Check sheet for the modelled part. Datum: model origin and axes. Units: mm. A direction names the side the tool comes from. Round coordinates to 2 decimals unless told otherwise and drop trailing zeros. Write each loop counter-clockwise with the first axis right and the second up, starting at its lowest first coordinate (ties: lowest second). Pieces come first, ordered by that corner, then holes. Notation, with made-up numbers: (8.5, 4.5) -> (48.5, 4.5) arc R27 ccw to (48.5, 43.5) -> close; hole circle Ø1 at (85.25, 15.5). An arc over 180 degrees is marked (long way). One line per item, written item: value. Start each with the question number.
Solid Edge part; units mm, degrees
sketch "Sketch1" plane through (0, 0, 0) normal (0, 0, 1) x (1, 0, 0)
  line L0 (-6.1009, 4.0673) -> (-6.5728, -3.2499)
  line L1 (-6.5728, -3.2499) -> (-0.4719, -7.3171)
  line L2 (-0.4719, -7.3171) -> (6.1009, -4.0673)
  line L3 (6.1009, -4.0673) -> (6.5728, 3.2499)
  line L4 (6.5728, 3.2499) -> (0.4719, 7.3171)
  line L5 (0.4719, 7.3171) -> (-6.1009, 4.0673)
extrude "Protrusion1" add sketch "Sketch1" against normal blind 225
sketch "Sketch2" plane through (0, 0, -2) normal (0, 0, 1) x (-0.8964, -0.4432, 0)
  circle A0 centre (0, 0) radius 5.5
  circle A1 centre (0, 0) radius 13.1424
extrude "ExtrudedCutout_1" cut sketch "Sketch2" against normal blind 2
sketch "Sketch3" plane through (0, 0, -223) normal (0, 0, -1) x (0.8964, 0.4432, 0)
  circle A0 centre (0, 0) radius 5.5
  circle A1 centre (0, 0) radius 13.1424
extrude "ExtrudedCutout_2" cut sketch "Sketch3" against normal blind 2
properties part number "BumbleB0197"
1. Release check for a two-part mould opening along Z. For faces 3 (the face through (-2.8, 5.7, -111)), 4 (the face through (-5, -3, -2)), 5 (the face through (5.435, 0.844, -222.014)), 6 (the face through (0, 0, 0)) record: +Z half, -Z half, draft (parallel to the pull), parting line (faces both ways), or undercut.
2. Cross-section at C-C (x = 2.75). Record the cut outline in (y, z), plus the area to 3 significant figures.
3. Depth check by flat-ended pin: pin 1 Ø6 at (x, z) = (-2.5, -150) entering from -Y; pin 2 Ø6 at (x, z) = (-3.5, -93) entering from +Y; pin 3 Ø6 at (x, z) = (4.5, -78.5) entering from +Y. Enter the tip coordinate at first touch or a pass-through.
4. Material ranges on probe 1 along Z at (x, y) = (5.75, 3); probe 2 along X at (y, z) = (-6, -154); probe 3 along X at (y, z) = (0.5, -81.5), recorded low to high.
5. Cross-section at A-A (z = -86). Record the cut outline in (x, y), plus the area to 3 significant figures.
6. Cross-section at B-B (y = 0). Record the cut outline in (x, z), plus the area to 3 significant figures.
7. Access from +Z, -Z, +X, -X, +Y, -Y to the whole of each face (thin tool, end or side, straight path). Record for faces 1 (the face through (2.8, -5.7, -111)), 2 (the face through (5, -3, -221)).
Working result:
1. face 3: draft
1. face 4: undercut
1. face 5: undercut
1. face 6: +Z half
2. outline: (-5.72, -225) -> (5.8, -225) -> (5.8, -223) -> (4.76, -223) -> (4.76, -221) -> (5.8, -221) -> (5.8, -4) -> (4.76, -4) -> (4.76, -2) -> (5.8, -2) -> (5.8, 0) -> (-5.72, 0) -> (-5.72, -2) -> (-4.76, -2) -> (-4.76, -4) -> (-5.72, -4) -> (-5.72, -221) -> (-4.76, -221) -> (-4.76, -223) -> (-5.72, -223) -> close
2. area: 2,580 mm^2
3. pin 1: stops at y = -7.32
3. pin 2: stops at y = 6.84
3. pin 3: stops at y = 6.63
4. probe 1: z = -225 to -223, -221 to -4, -2 to 0
4. probe 2: x = -2.45 to 2.19
4. probe 3: x = -6.33 to 6.4
5. outline: (-6.57, -3.25) -> (-0.47, -7.32) -> (6.1, -4.07) -> (6.57, 3.25) -> (0.47, 7.32) -> (-6.1, 4.07) -> close
5. area: 140 mm^2
6. outline: (-6.36, -225) -> (6.36, -225) -> (6.36, -223) -> (5.5, -223) -> (5.5, -221) -> (6.36, -221) -> (6.36, -4) -> (5.5, -4) -> (5.5, -2) -> (6.36, -2) -> (6.36, 0) -> (-6.36, 0) -> (-6.36, -2) -> (-5.5, -2) -> (-5.5, -4) -> (-6.36, -4) -> (-6.36, -221) -> (-5.5, -221) -> (-5.5, -223) -> (-6.36, -223) -> close
6. area: 2,860 mm^2
7. face 1: +Z, -Z, +X, -Y
7. face 2: none
